Source: CAD feature listing. Evaluate the final solid. Frame: model axes, mm. A direction names the side the tool comes from. Round coordinates to 2 decimals unless told otherwise and drop trailing zeros. Write each loop counter-clockwise with the first axis right and the second up, starting at its lowest first coordinate (ties: lowest second). Pieces come first, ordered by that corner, then holes. Notation, with made-up numbers: M 18,69 L 63,69 A18 ccw 63,92 Z; hole C 65,1.25 d6. An arc over 180 degrees is marked long. Answer in a Markdown table with one row per item.
from build123d import *

# Parameters (mm, degrees)
BOSS_EXTRUDE2_DEPTH = 2
BOSS_EXTRUDE3_DEPTH = 36


with BuildPart() as part:
    # Sketch1 → Boss-Extrude2 (new body)
    with BuildSketch(Plane.XY):
        with BuildLine():
            ThreePointArc((36.77383834, 0.897309378), (30.841544287, 5.867048301), (34.547643901, 12.660813336))
            ThreePointArc((34.547643901, 12.660813336), (38.439664011, 25.419866138), (25.151092425, 26.583959838))
            ThreePointArc((25.151092425, 26.583959838), (15.658221947, 25.240839631), (12.033396672, 34.116604585))
            ThreePointArc((12.033396672, 34.116604585), (-0.388796102, 49.993952041), (-11.79974319, 33.374947194))
            ThreePointArc((-11.79974319, 33.374947194), (-15.701881175, 19.773765205), (-29.82628778, 18.925254505))
            ThreePointArc((-29.82628778, 18.925254505), (-49.422493782, 9.994241781), (-33.625891529, -4.642753649))
            ThreePointArc((-33.625891529, -4.642753649), (-13.793191326, -11.35592194), (-11.294565378, -32.144368111))
            ThreePointArc((-11.294565378, -32.144368111), (-0.472558297, -49.991064352), (11.666927416, -33.013040598))
            ThreePointArc((11.666927416, -33.013040598), (15.7550057, -16.875289061), (32.331827923, -15.342848629))
            ThreePointArc((32.331827923, -15.342848629), (45.072719303, -10.100170445), (36.77383834, 0.897309378))
        make_face()
    extrude(amount=BOSS_EXTRUDE2_DEPTH)

    # Sketch2 → Boss-Extrude3 (add)
    with BuildSketch(Plane.XY.offset(2)):
        with BuildLine():
            ThreePointArc((34.547643726, 12.660813265), (30.841544291, 5.867048278), (36.773838199, 0.89730938))
            ThreePointArc((36.773838199, 0.89730938), (45.072719321, -10.100170381), (32.331827916, -15.342848625))
            ThreePointArc((32.331827916, -15.342848625), (15.755005651, -16.875289103), (11.666927459, -33.013040709))
            ThreePointArc((11.666927459, -33.013040709), (-0.472558319, -49.991064352), (-11.29456541, -32.14436818))
            ThreePointArc((-11.29456541, -32.14436818), (-13.793191238, -11.355922049), (-33.62589133, -4.642753601))
            ThreePointArc((-33.62589133, -4.642753601), (-49.422493786, 9.994241754), (-29.826287652, 18.925254425))
            ThreePointArc((-29.826287652, 18.925254425), (-15.701881135, 19.773765237), (-11.799743174, 33.374947148))
            ThreePointArc((-11.799743174, 33.374947148), (-0.388796168, 49.993952038), (12.033396695, 34.116604666))
            ThreePointArc((12.033396695, 34.116604666), (15.65822203, 25.240839584), (25.151092616, 26.583960036))
            ThreePointArc((25.151092616, 26.583960036), (38.439664141, 25.419865946), (34.547643726, 12.660813265))
        make_face()
        with BuildLine():
            ThreePointArc((-31.408898966, 16.376658454), (-13.825543659, 17.432962452), (-8.967804812, 34.364959833))
            ThreePointArc((-8.967804812, 34.364959833), (-0.295485088, 46.995403549), (9.145381488, 34.928619546))
            ThreePointArc((9.145381488, 34.928619546), (14.164303925, 22.639261467), (27.308104459, 24.498942072))
            ThreePointArc((27.308104459, 24.498942072), (35.952987853, 23.741640383), (33.421033039, 15.4412356))
            ThreePointArc((33.421033039, 15.4412356), (27.893864073, 5.309211984), (36.741114762, -2.102512145))
            ThreePointArc((36.741114762, -2.102512145), (42.179011051, -9.308682891), (33.830458389, -12.743982198))
            ThreePointArc((33.830458389, -12.743982198), (13.805341223, -14.595199495), (8.866864868, -34.089910939))
            ThreePointArc((8.866864868, -34.089910939), (-0.359144322, -46.993208907), (-8.583869712, -33.429719817))
            ThreePointArc((-8.583869712, -33.429719817), (-11.464280061, -9.464844913), (-34.327373037, -1.725919116))
            ThreePointArc((-34.327373037, -1.725919116), (-46.460737086, 9.516751182), (-31.408898966, 16.376658454))
        make_face(mode=Mode.SUBTRACT)
    extrude(amount=BOSS_EXTRUDE3_DEPTH)


solid = part.part
Q1. Pull-direction query (X, two-part tool) for faces 1 (the cylindrical face through (13.99, 22.74, 19.75)), 2 (the flat face through (-3, 1, 0)); classes: pulls with the +X half, pulls with the -X half, needs draft (parallel to the pull), parting line crosses it, or undercut.
Solutions:
| item | result |
|---|---|
| face 1 | undercut |
| face 2 | needs draft |
Q2. Material intervals for probe 1 along X at (y, z) = (-37.5, 25); probe 2 along X at (y, z) = (5, 6); probe 3 along Z at (x, y) = (-23.5, 2), sorted ascending.
Solutions:
| item | result |
|---|---|
| probe 1 | x = -12.5 to -9.5, 9.5 to 12.5 |
| probe 2 | x = -49.25 to -46.14, 27.96 to 31.07 |
| probe 3 | z = 0 to 2 |
Q3. Section B-B (y = -37.5). Return loops of the section in (x, z).
Solutions:
| item | result |
|---|---|
| outline | M -12.5,0 L 12.5,0 L 12.5,38 L 9.5,38 L 9.5,2 L -9.5,2 L -9.5,38 L -12.5,38 Z |
Q4. Access query for faces 3 (the cylindrical face through (42.216, -9.168, 19.748)), 4 (the flat face through (-12, -11, 38)). Directions: +Z, -Z, +X, -X, +Y, -Y. A direction counts if a zero-diameter tool reaches every point of the face in a straight line with its end or side. Return the directions, or none.
Solutions:
| item | result |
|---|---|
| face 3 | +Z |
| face 4 | +Z, +X, -X, +Y, -Y |
Q5. Section A-A (x = 0). Return loops of the section in (y, z), and give its area (3 significant figures).
Solutions:
| item | result |
|---|---|
| outline | M -50,0 L 50,0 L 50,38 L 47,38 L 47,2 L -47,2 L -47,38 L -50,38 Z |
| area | 416 mm2 |
Q6. Section C-C (z = 5). Return loops of the section in (x, y), and give its area (3 significant figures).
Solutions:
| item | result |
|---|---|
| outline | M -33.63,-4.64 A19.63 cw -11.29,-32.14 A12.5 ccw long 11.67,-33.01 A14.42 cw 32.33,-15.34 A8.7 ccw long 36.77,0.9 A6.11 cw 34.55,12.66 A8.58 ccw long 25.15,26.58 A7.8 cw 12.03,34.12 A12.5 ccw long -11.8,33.37 A12.25 cw -29.83,18.93 A12.94 ccw long Z; hole M -34.33,-1.73 A22.63 cw -8.58,-33.43 A9.5 ccw long 8.87,-34.09 A17.42 cw 33.83,-12.74 A5.7 ccw long 36.74,-2.1 A9.11 cw 33.42,15.44 A5.58 ccw long 27.31,24.5 A10.8 cw 9.15,34.93 A9.5 ccw long -8.97,34.36 A15.25 cw -31.41,16.38 A9.94 ccw long Z |
| area | 1,040 mm2 |
Q7. Contact query for flat-ended pins moving along their axis: pin 1 Ø12 at (y, z) = (-34, 10) entering from +X; pin 2 Ø5 at (x, z) = (21.5, 30) entering from +Y; pin 3 Ø5 at (x, z) = (12, 7.5) entering from -Y. Output: stop coordinate, or through.
Solutions:
| item | result |
|---|---|
| pin 1 | stops at x = 12.5 |
| pin 2 | stops at y = 25.6 |
| pin 3 | stops at y = -45.62 |
